Here's how the part is built. I have some questions about the finished solid (model axes, mm). Face numbers are marked on the shaded views. A direction names the side the tool comes from. Coordinates: 2 decimals unless noted, no trailing zeros. Write each loop counter-clockwise with the first axis right and the second up, starting at its lowest first coordinate (ties: lowest second). Pieces come first, ordered by that corner, then holes. Notation, with made-up numbers: M 18.25,16.25 L 38.25,16.25 A21 cw 38.25,33.25 Z; hole C -29.5,-23.5 d11. An arc over 180 degrees is marked long. Use one line per item in the form item = value. Start each with the question number.
1. I want a section at A-A, the plane x = -46.5. List the corners of the cut face in (y, z) for me.
2. I want a section at B-B, the plane y = 7. List the corners of the cut face in (x, z) for me, plus the area to 3 significant figures.
3. On a 3-axis mill with a long thin cutter (end or side, diameter ignored), from which of +Z, -Z, +X, -X, +Y, -Y can I reach the whole of each face in a straight line? I mean the marked faces 1 and 2. Say none if no direction works.
4. Please list where these lines run through material, in increasing order: line 1 along Z through (x, y) = (-47, 11); line 2 along X through (y, z) = (10.25, 4.75); line 3 along X through (y, z) = (9.5, -4). Write a range as [from, to].
5. I want a section at C-C, the plane z = 1.25. List the corners of the cut face in (x, y) for me, plus the area to 3 significant figures.
6. I want a section at D-D, the plane y = 14.25. List the corners of the cut face in (x, z) for me.
7. I'm going to push flat-ended pins straight in: pin 1 Ø2.5 at (y, z) = (10, -0.5) entering from -X; pin 2 Ø4.5 at (y, z) = (10, 0) entering from +X; pin 3 Ø4.5 at (x, y) = (-50.92, 10.53) entering from +Z. Where does each tip first touch, or does it pass through?
8. Thinking about a two-plate mould opening in Z: for the marked faces 3, 4, 5 and 6, which applies, released by +Z, released by -Z, zero draft, split by the parting line, or undercut?
from build123d import *

# Parameters (mm, degrees)
EXTRUDE_1_DEPTH     = 6
SKETCH_2_R          = 2.5
SKETCH_2_R_2        = 1.5
CUT_EXTRUDE_1_DEPTH = 12
CUT_EXTRUDE_2_DEPTH = 4.5


with BuildPart() as part:
    # 草图1 → 凸台-拉伸1 (new, symmetric)
    with BuildSketch(Plane.XY):
        with BuildLine():
            Line((-50.916030534, 15.534351145), (39.083969466, 15.534351145))
            ThreePointArc((39.083969466, 15.534351145), (44.083969466, 10.534351145), (39.083969466, 5.534351145))
            Line((39.083969466, 5.534351145), (-50.916030534, 5.534351145))
            ThreePointArc((-50.916030534, 5.534351145), (-55.916030534, 10.534351145), (-50.916030534, 15.534351145))
        make_face()
    extrude(amount=EXTRUDE_1_DEPTH, both=True)

    # 草图2 → 切除-拉伸1 (cut)
    with BuildSketch(Plane.XY.offset(6)):
        with Locations((-50.916030534, 10.534351145)):
            Circle(SKETCH_2_R)
        with Locations((39.083969466, 10.534351145)):
            Circle(SKETCH_2_R_2)
    extrude(amount=-CUT_EXTRUDE_1_DEPTH, mode=Mode.SUBTRACT)

    # 草图3 → 切除-拉伸2 (cut, symmetric)
    with BuildSketch(Plane.XY):
        with BuildLine():
            Line((39.083969466, 15.534351145), (13.083969466, 15.534351145))
            Line((13.083969466, 15.534351145), (13.083969466, 5.534351145))
            Line((13.083969466, 5.534351145), (39.083969466, 5.534351145))
            ThreePointArc((39.083969466, 5.534351145), (44.083969466, 10.534351145), (39.083969466, 15.534351145))
        make_face()
        with BuildLine():
            Line((-50.916030534, 15.534351145), (-44.916030534, 15.534351145))
            Line((-44.916030534, 15.534351145), (-44.916030534, 5.534351145))
            Line((-44.916030534, 5.534351145), (-50.916030534, 5.534351145))
            ThreePointArc((-50.916030534, 5.534351145), (-55.916030534, 10.534351145), (-50.916030534, 15.534351145))
        make_face()
    extrude(amount=CUT_EXTRUDE_2_DEPTH, both=True, mode=Mode.SUBTRACT)


solid = part.part
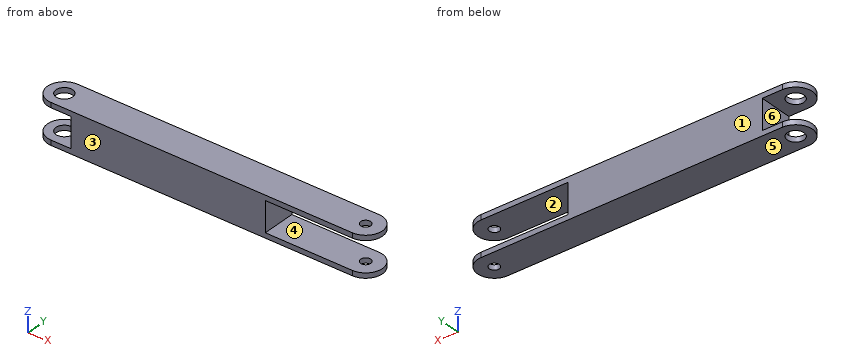
Answer list:
q1.outline = M 5.53,-6 L 15.53,-6 L 15.53,-4.5 L 5.53,-4.5 Z; M 5.53,4.5 L 15.53,4.5 L 15.53,6 L 5.53,6 Z
q2.outline = M -54.45,-6 L 42.62,-6 L 42.62,-4.5 L 13.08,-4.5 L 13.08,4.5 L 42.62,4.5 L 42.62,6 L -54.45,6 L -54.45,4.5 L -44.92,4.5 L -44.92,-4.5 L -54.45,-4.5 Z
q2.area = 813 mm²
q3.face_1 = +Z, -Z, +X, -X, +Y
q3.face_2 = +X, +Y, -Y
q4.line_1 = [-6, -4.5], [4.5, 6]
q4.line_2 = [-55.91, -53.4], [-48.43, 37.61], [40.56, 44.08]
q4.line_3 = [-44.92, 13.08]
q5.outline = M -44.92,5.53 L 13.08,5.53 L 13.08,15.53 L -44.92,15.53 Z
q5.area = 580 mm²
q6.outline = M -54.26,-6 L 42.43,-6 L 42.43,-4.5 L 13.08,-4.5 L 13.08,4.5 L 42.43,4.5 L 42.43,6 L -54.26,6 L -54.26,4.5 L -44.92,4.5 L -44.92,-4.5 L -54.26,-4.5 Z
q7.pin_1 = -44.92
q7.pin_2 = 13.08
q7.pin_3 = through
q8.face_3 = zero draft
q8.face_4 = undercut
q8.face_5 = released by -Z
q8.face_6 = undercut
